Verification items for the finished model (mm, model axes). A direction names the side the tool comes from. Give positions to 0.01 mm unless a question says otherwise; leave off trailing zeros. Write each loop counter-clockwise with the first axis right and the second up, starting at its lowest first coordinate (ties: lowest second). Pieces come first, ordered by that corner, then holes.
from build123d import *

# Parameters (mm, degrees)
SKETCH1_W           = 32
SKETCH1_H           = 40
SKETCH1_R           = 1.5
SKETCH1_R_2         = 1
SKETCH1_W_2         = 11.5
SKETCH1_H_2         = 22
BOSS_EXTRUDE1_DEPTH = 2.5
FILLET1_R           = 5


with BuildPart() as part:
    # Sketch1 → Boss-Extrude1 (new body)
    with BuildSketch(Plane(origin=(0, 0, 0), x_dir=(1, 0, 0), z_dir=(0, 1, 0))):
        Rectangle(SKETCH1_W, SKETCH1_H)
        with Locations(Location((11, 15, 0), (0, 0, 270))):
            Circle(SKETCH1_R, mode=Mode.SUBTRACT)
        with Locations(Location((11, 0, 0), (0, 0, 270))):
            Circle(SKETCH1_R, mode=Mode.SUBTRACT)
        with Locations(Location((11, -15, 0), (0, 0, 270))):
            Circle(SKETCH1_R, mode=Mode.SUBTRACT)
        with Locations(Location((-7.25, -14, 0), (0, 0, 270))):
            Circle(SKETCH1_R_2, mode=Mode.SUBTRACT)
        with Locations(Location((-7.25, 14, 0), (0, 0, 90))):
            Circle(SKETCH1_R_2, mode=Mode.SUBTRACT)
        with Locations((-7.25, 0)):
            Rectangle(SKETCH1_W_2, SKETCH1_H_2, mode=Mode.SUBTRACT)
    extrude(amount=BOSS_EXTRUDE1_DEPTH)

    # Fillet1
    fillet1_edges = [part.edges().sort_by_distance(p)[0] for p in [
        (-16, 1.25, -20),
        (16, 1.25, -20),
        (16, 1.25, 20),
        (-16, 1.25, 20),
    ]]
    fillet(fillet1_edges, radius=FILLET1_R)


solid = part.part
Item 1: Sectioned sample at A-A on z = -10. Record the cut outline in (x, y), then the cut area to 4 significant figures.
Answer key:
outline: (-16, 0) - (-13, 0) - (-13, 2.5) - (-16, 2.5) - close; (-1.5, 0) - (16, 0) - (16, 2.5) - (-1.5, 2.5) - close
area: 51.25 mm2
Item 2: Sectioned sample at C-C on y = 2.1. Record the cut outline in (x, z).
Answer key:
outline: (-16, -15) arc R5 ccw to (-11, -20) - (11, -20) arc R5 ccw to (16, -15) - (16, 15) arc R5 ccw to (11, 20) - (-11, 20) arc R5 ccw to (-16, 15) - close; hole (-13, -11) - (-1.5, -11) - (-1.5, 11) - (-13, 11) - close; hole circle Ø2 at (-7.25, -14); hole circle Ø2 at (-7.25, 14); hole circle Ø3 at (11, -15); hole circle Ø3 at (11, 0); hole circle Ø3 at (11, 15)
Item 3: Scan lines: line 1 along X through (y, z) = (1.9, 4.5); line 2 along X through (y, z) = (0.6, -14); line 3 along Z through (x, y) = (-6, 2). Record each from-to range of solid material in increasing order.
Answer key:
line 1: x = -16 to -13, -1.5 to 16
line 2: x = -16 to -8.25, -6.25 to 9.88, 12.12 to 16
line 3: z = -20 to -11, 11 to 20
Item 4: Sectioned sample at B-B on x = -7.25. Record the cut outline in (y, z), then the cut area to 3 significant figures.
Answer key:
outline: (0, -20) - (2.5, -20) - (2.5, -15) - (0, -15) - close; (0, -13) - (2.5, -13) - (2.5, -11) - (0, -11) - close; (0, 11) - (2.5, 11) - (2.5, 13) - (0, 13) - close; (0, 15) - (2.5, 15) - (2.5, 20) - (0, 20) - close
area: 35.0 mm2
Item 5: Sectioned sample at D-D on z = 1. Record the cut outline in (x, y), then the cut area to 3 significant figures.
Answer key:
outline: (-16, 0) - (-13, 0) - (-13, 2.5) - (-16, 2.5) - close; (-1.5, 0) - (9.88, 0) - (9.88, 2.5) - (-1.5, 2.5) - close; (12.12, 0) - (16, 0) - (16, 2.5) - (12.12, 2.5) - close
area: 45.7 mm2
Item 6: Release check for a two-part mould opening along X. For faces 3 (the face through (16, 1, 0)), 4 (the face through (-1.5, 1, 0)), 5 (the face through (0, 1, 20)) record: released by +X, released by -X, zero draft, split by the parting line, or undercut.
Answer key:
face 3: released by +X
face 4: undercut
face 5: zero draft
Item 7: Set-up check for faces 1 (the face through (-7, 1, -11)), 2 (the face through (0, 0, 0)): record each of +Z, -Z, +X, -X, +Y, -Y from which the full face is reachable in a straight line by a thin tool's end or side.
Answer key:
face 1: +Y, -Y
face 2: +Z, -Z, +X, -X, -Y
